Here's how the part is built. I have some questions about the finished solid (model axes, mm). A direction names the side the tool comes from. Round coordinates to 2 decimals unless told otherwise and drop trailing zeros. Loops run counter-clockwise (first coordinate to the right, second up) from the corner with the lowest first, then second, coordinate; pieces in that order, holes last. Notation, with made-up numbers: M -11.75,-37.5 L 25.25,-37.5 A5 cw 25.25,-31.5 Z; hole C 13,65.5 d3. An arc over 180 degrees is marked long. Put each result on its own line as item: value. Start each with the question number.
```python
from build123d import *

# Parameters (mm, degrees)
F0_W     = 12.7
F0_H     = 12.7
F1_DEPTH = 100
F2_W     = 12.7
F2_H     = 52.3
F2_H_2   = 12.7
F2_W_2   = 52.3
F3_DEPTH = 2.5
F4_R     = 5.08


with BuildPart() as f1:
    # F0 (on Top) → F1 (new body)
    with BuildSketch(Plane.XY):
        with Locations((-32.5, 32.5)):
            Rectangle(F0_W, F0_H)
    extrude(amount=F1_DEPTH)



with BuildPart() as f1b:
    # F0 (on Top) → F1, piece 2 (new body)
    with BuildSketch(Plane.XY):
        with Locations((32.5, 32.5)):
            Rectangle(F0_W, F0_H)
    extrude(amount=F1_DEPTH)


with BuildPart() as f1c:
    # F0 (on Top) → F1, piece 3 (new body)
    with BuildSketch(Plane.XY):
        with Locations((32.5, -32.5)):
            Rectangle(F0_W, F0_H)
    extrude(amount=F1_DEPTH)


with BuildPart() as f1d:
    # F0 (on Top) → F1, piece 4 (new body)
    with BuildSketch(Plane.XY):
        with Locations((-32.5, -32.5)):
            Rectangle(F0_W, F0_H)
    extrude(amount=F1_DEPTH)


with BuildPart() as f1_1:
    add(f1.part)

    add(f1b.part)  # F3 merges F1b

    add(f1c.part)  # F3 merges F1c

    add(f1d.part)  # F3 merges F1d
    # F2 (on face) → F3 (join)
    with BuildSketch(Plane.XY.offset(100)):
        with Locations((-32.5, 0)):
            Rectangle(F2_W, F2_H)
        with Locations((-32.5, 32.5)):
            Rectangle(F2_W, F2_H_2)
        with Locations((0, 32.5)):
            Rectangle(F2_W_2, F2_H_2)
        with Locations((32.5, 32.5)):
            Rectangle(F2_W, F2_H_2)
        with Locations((32.5, 0)):
            Rectangle(F2_W, F2_H)
        with Locations((32.5, -32.5)):
            Rectangle(F2_W, F2_H_2)
        with Locations((0, -32.5)):
            Rectangle(F2_W_2, F2_H_2)
        with Locations((-32.5, -32.5)):
            Rectangle(F2_W, F2_H_2)
    extrude(amount=F3_DEPTH)

    # F4
    f4_edges = [f1_1.edges().sort_by_distance(p)[0] for p in [
        (38.85, -38.85, 51.25),
        (38.85, 38.85, 51.25),
        (-38.85, 38.85, 51.25),
        (-38.85, -38.85, 51.25),
    ]]
    fillet(f4_edges, radius=F4_R)


solid = f1_1.part
```
1) Suppose I cut it at C-C (z = 36.5). Write out the boundary of the cut face in (x, y), plus the area to 3 significant figures.
2) I'm going to push a flat-ended pin straight in: P1, Ø14, axis at x = 8.5, y = -32, coming from the -Z side. Where does the tip first touch, or does it pass through?
3) If I drill on probe 1 along Y at (x, z) = (-32, 92.5); probe 2 along X at (y, z) = (-34, 5.5); probe 3 along Z at (x, y) = (19.5, 27), over which ranges is the centre line in solid material (lowest first)? Write a range as from..to.
4) Suppose I cut it at D-D (x = 30). Write out the boundary of the cut face in (y, z).
5) Suppose I cut it at A-A (y = -3). Write out the boundary of the cut face in (x, z).
6) On a 3-axis mill with a long thin cutter (end or side, diameter ignored), from which of +Z, -Z, +X, -X, +Y, -Y can I reach the whole of each face in a straight line? I mean faces 1 (the face through (-37.401, -37.322, 51.968)), 2 (the face through (-26.15, 0, 101)), 3 (the face through (32, 0, 100)), 4 (the face through (26.15, -33, 49)). Say none if no direction works.
7) If we mould it in two halves opening along X, with no side actions, what happens to faces 5 (the face through (26.15, 32, 49)), 6 (the face through (37.401, -37.322, 51.968)), 7 (the face through (-38.85, 28, 59))? For each: pulls with the +X half, pulls with the -X half, needs draft (parallel to the pull), parting line crosses it, or undercut.
Results are:
1. outline: M -38.85,-33.77 A5.08 ccw -33.77,-38.85 L -26.15,-38.85 L -26.15,-26.15 L -38.85,-26.15 Z; M -38.85,26.15 L -26.15,26.15 L -26.15,38.85 L -33.77,38.85 A5.08 ccw -38.85,33.77 Z; M 26.15,-38.85 L 33.77,-38.85 A5.08 ccw 38.85,-33.77 L 38.85,-26.15 L 26.15,-26.15 Z; M 26.15,26.15 L 38.85,26.15 L 38.85,33.77 A5.08 ccw 33.77,38.85 L 26.15,38.85 Z
1. area: 623 mm²
2. P1: z = 100
3. probe 1: -38.85..-26.15, 26.15..38.85
3. probe 2: -38.84..-26.15, 26.15..38.84
3. probe 3: 100..102.5
4. outline: M -38.85,0 L -26.15,0 L -26.15,100 L 26.15,100 L 26.15,0 L 38.85,0 L 38.85,102.5 L -38.85,102.5 Z
5. outline: M -38.85,100 L -26.15,100 L -26.15,102.5 L -38.85,102.5 Z; M 26.15,100 L 38.85,100 L 38.85,102.5 L 26.15,102.5 Z
6. face 1: +Z, -Z, -X, -Y
6. face 2: +Z, -Z
6. face 3: -Z, +X, -X
6. face 4: -Z, +Y, -Y
7. face 5: undercut
7. face 6: pulls with the +X half
7. face 7: pulls with the -X half
